Check sheet for the modelled part. Datum: model origin and axes. Units: mm. Face numbers are marked on the shaded views. A direction names the side the tool comes from. Give positions to 0.01 mm unless a question says otherwise; leave off trailing zeros. Order: outer loops, then holes, each group sorted by start corner. A loop starts at its lowest first (then second) coordinate and runs counter-clockwise, first axis right, second up.
```python
from build123d import *

# Parameters (mm, degrees)
PAD_DEPTH            = 22
POCKET_DEPTH         = 20
POCKET001_DEPTH      = 10
SKETCH003_R          = 1
POCKET002_DEPTH      = 16.25
POCKET002_DEPTH_BACK = -16.25
SKETCH004_R          = 1.1
PAD001_DEPTH         = 9
SKETCH005_R          = 1
POCKET003_DEPTH      = 5


with BuildPart() as part:
    # Sketch → Pad (new body)
    with BuildSketch(Plane.XY):
        Polygon((0, -17.960512), (17.960512, 0), (0, 17.960512), (-17.960512, 0), align=None)
    extrude(amount=PAD_DEPTH)

    # Sketch001 (on Face6 of Pad) → Pocket (cut)
    with BuildSketch(Plane.XY.offset(22)):
        Polygon((0, 14.849242), (-14.849242, 0), (0, -14.849242), (14.849242, 0), align=None)
    extrude(amount=-POCKET_DEPTH, mode=Mode.SUBTRACT)

    # Sketch002 (on Face5 of Pocket) → Pocket001 (cut)
    with BuildSketch(Plane.XY.offset(22)):
        Polygon((-3.11127, 14.849242), (-17.960512, 0), (-3.11127, -14.849242), (0, -14.849242), (-14.849242, 0), (0, 14.849242), align=None)
    pocket001 = extrude(amount=-POCKET001_DEPTH, mode=Mode.SUBTRACT)

    # Mirrored: Pocket001 across YZ
    add(pocket001.mirror(Plane.YZ), mode=Mode.SUBTRACT)

    # Sketch003 → Pocket002 (cut, two sides)
    with BuildSketch(Plane.XZ) as pocket002_sk:
        with Locations((0, 19.622342)):
            Circle(SKETCH003_R)
    extrude(amount=-POCKET002_DEPTH, mode=Mode.SUBTRACT)
    extrude(pocket002_sk.sketch, amount=-POCKET002_DEPTH_BACK, mode=Mode.SUBTRACT)

    # Sketch004 (on Face15 of Pocket002) → Pad001 (join)
    with BuildSketch(Plane.XY.offset(12)):
        with Locations((8.202439, 8.202439)):
            Circle(SKETCH004_R)
    pad001 = extrude(amount=PAD001_DEPTH)

    # Mirrored001: Pad001 across YZ
    add(pad001.mirror(Plane.YZ))

    # Sketch005 (on Face21 of Mirrored001) → Pocket003 (cut)
    with BuildSketch(Plane.XY.offset(2)):
        with Locations((-11, 0)):
            Circle(SKETCH005_R)
        with Locations((11, 0)):
            Circle(SKETCH005_R)
    extrude(amount=-POCKET003_DEPTH, mode=Mode.SUBTRACT)


solid = part.part
```
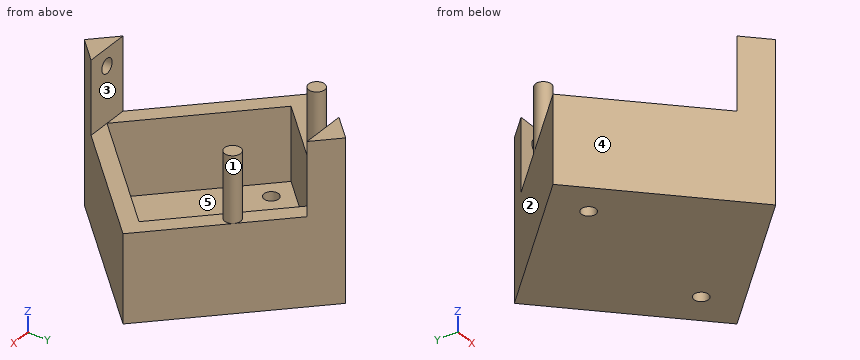
(1) Go/stop test with flat-tipped pins: P1, Ø1.2, axis at x = 0, z = 19.62, coming from the -Y side; P2, Ø10, axis at x = 9.5, y = 8.5, coming from the +Z side; P3, Ø2.5, axis at x = 11, y = 0, coming from the -Z side; P4, Ø3, axis at x = 0, z = 19.62, coming from the +Y side. Record where each tip stops, or that it passes through.
(2) Sectioned sample at A-A (z = 10.5). Enter the section's corners in (x, y), plus the area to 3 significant figures.
(3) Sectioned sample at D-D (z = 15). Enter the section's corners in (x, y).
(4) Sectioned sample at C-C (y = -0.5). Enter the section's corners in (x, z), plus the area to 3 significant figures.
(5) Release check for a two-part mould opening along X. For the marked faces 3, 4 and 5 record: released by +X, released by -X, zero draft, split by the parting line, or undercut.
(6) Thickness scan on L1, parallel to Z at x = 0, y = 15.6; L2, parallel to Z at x = -11, y = 5; L3, parallel to Y at x = -10.5, z = 9. Record the ranges inside material, lowest first.
(7) Tool access check on the marked faces 1 and 2. Record the directions out of +Z, -Z, +X, -X, +Y, -Y that give a thin tool (end or side, any length) a straight path to the whole face; none if there is none.
(8) Sectioned sample at B-B (x = -11). Enter the section's corners in (y, z), plus the area to 3 significant figures.
Values follow:
1. P1: stops at y = -17.96
1. P2: stops at z = 21
1. P3: stops at z = 0
1. P4: stops at y = 17.96
2. outline: (-17.96, 0) - (0, -17.96) - (17.96, 0) - (0, 17.96) - close; hole (-14.85, 0) - (0, -14.85) - (14.85, 0) - (0, 14.85) - close
2. area: 204 mm2
3. outline: circle Ø2.2 at (-8.2, 8.2); (-3.11, -14.85) - (0, -17.96) - (3.11, -14.85) - close; (-3.11, 14.85) - (3.11, 14.85) - (0, 17.96) - close; circle Ø2.2 at (8.2, 8.2)
4. outline: (-17.46, 0) - (-11.87, 0) - (-11.87, 2) - (-14.35, 2) - (-14.35, 12) - (-17.46, 12) - close; (-10.13, 0) - (10.13, 0) - (10.13, 2) - (-10.13, 2) - close; (11.87, 0) - (17.46, 0) - (17.46, 12) - (14.35, 12) - (14.35, 2) - (11.87, 2) - close
4. area: 125 mm2
5. face 3: zero draft
5. face 4: released by -X
5. face 5: undercut
6. L1: z = 0 to 18.62, 20.62 to 22
6. L2: z = 0 to 12
6. L3: y = -7.46 to -4.35, 4.35 to 7.46
7. face 1: +Z
7. face 2: +Z, -Z, -X, +Y
8. outline: (-6.96, 0) - (-1, 0) - (-1, 2) - (-3.85, 2) - (-3.85, 12) - (-6.96, 12) - close; (1, 0) - (6.96, 0) - (6.96, 12) - (3.85, 12) - (3.85, 2) - (1, 2) - close
8. area: 86.1 mm2
